from build123d import *

# Parameters (mm, degrees)
SKETCH1_R           = 79.375
SKETCH1_R_2         = 66.675
SKETCH1_R_3         = 1.4224
BOSS_EXTRUDE1_DEPTH = 3.048
SKETCH2_R           = 1.4224
BOSS_EXTRUDE2_DEPTH = 3.048


with BuildPart() as part:
    # Sketch1 → Boss-Extrude1 (new body)
    with BuildSketch(Plane(origin=(0, 0, 0), x_dir=(1, 0, 0), z_dir=(0, 1, 0))):
        with Locations(Location((0, 0, 0), (0, 0, 90))):
            Circle(SKETCH1_R)
        with Locations(Location((0, 0, 0), (0, 0, 90))):
            Circle(SKETCH1_R_2, mode=Mode.SUBTRACT)
        with Locations(Location((0, 73.025, 0), (0, 0, 90))):
            Circle(SKETCH1_R_3, mode=Mode.SUBTRACT)
        with Locations(Location((27.945457648, 67.466302862, 0), (0, 0, 90))):
            Circle(SKETCH1_R_3, mode=Mode.SUBTRACT)
        with Locations(Location((51.636472696, 51.636472696, 0), (0, 0, 90))):
            Circle(SKETCH1_R_3, mode=Mode.SUBTRACT)
        with Locations(Location((67.466302862, 27.945457648, 0), (0, 0, 90))):
            Circle(SKETCH1_R_3, mode=Mode.SUBTRACT)
        with Locations(Location((73.025, 0, 0), (0, 0, 90))):
            Circle(SKETCH1_R_3, mode=Mode.SUBTRACT)
        with Locations(Location((67.466302862, -27.945457648, 0), (0, 0, 90))):
            Circle(SKETCH1_R_3, mode=Mode.SUBTRACT)
        with Locations(Location((51.636472696, -51.636472696, 0), (0, 0, 90))):
            Circle(SKETCH1_R_3, mode=Mode.SUBTRACT)
        with Locations(Location((27.945457648, -67.466302862, 0), (0, 0, 90))):
            Circle(SKETCH1_R_3, mode=Mode.SUBTRACT)
        with Locations(Location((0, -73.025, 0), (0, 0, 90))):
            Circle(SKETCH1_R_3, mode=Mode.SUBTRACT)
        with Locations(Location((-27.945457648, -67.466302862, 0), (0, 0, 90))):
            Circle(SKETCH1_R_3, mode=Mode.SUBTRACT)
        with Locations(Location((-51.636472696, -51.636472696, 0), (0, 0, 90))):
            Circle(SKETCH1_R_3, mode=Mode.SUBTRACT)
        with Locations(Location((-67.466302862, -27.945457648, 0), (0, 0, 90))):
            Circle(SKETCH1_R_3, mode=Mode.SUBTRACT)
        with Locations(Location((-73.025, 0, 0), (0, 0, 90))):
            Circle(SKETCH1_R_3, mode=Mode.SUBTRACT)
        with Locations(Location((-67.466302862, 27.945457648, 0), (0, 0, 90))):
            Circle(SKETCH1_R_3, mode=Mode.SUBTRACT)
        with Locations(Location((-51.636472696, 51.636472696, 0), (0, 0, 90))):
            Circle(SKETCH1_R_3, mode=Mode.SUBTRACT)
        with Locations(Location((-27.945457648, 67.466302862, 0), (0, 0, 90))):
            Circle(SKETCH1_R_3, mode=Mode.SUBTRACT)
    extrude(amount=BOSS_EXTRUDE1_DEPTH)

    # Sketch2 → Boss-Extrude2 (add)
    with BuildSketch(Plane(origin=(0, 3.048, 0), x_dir=(1, 0, 0), z_dir=(0, 1, 0))):
        with BuildLine():
            Line((-15.494, 3.175), (-15.494, 27.813))
            ThreePointArc((-15.494, 27.813), (-12.319, 30.988), (-15.494, 34.163))
            Line((-15.494, 34.163), (-15.494, 58.801))
            ThreePointArc((-15.494, 58.801), (-13.24893597, 59.73093597), (-12.319, 61.976))
            Line((-12.319, 61.976), (-12.319, 65.527077334))
            ThreePointArc((-12.319, 65.527077334), (-17.128346163, 64.437375666), (-21.844, 62.995200524))
            Line((-21.844, 62.995200524), (-21.844, -62.995200524))
            ThreePointArc((-21.844, -62.995200524), (-17.128346163, -64.437375666), (-12.319, -65.527077334))
            Line((-12.319, -65.527077334), (-12.319, -61.976))
            ThreePointArc((-12.319, -61.976), (-13.24893597, -59.73093597), (-15.494, -58.801))
            Line((-15.494, -58.801), (-15.494, -34.163))
            ThreePointArc((-15.494, -34.163), (-12.319, -30.988), (-15.494, -27.813))
            Line((-15.494, -27.813), (-15.494, -3.175))
            ThreePointArc((-15.494, -3.175), (-12.319, 0), (-15.494, 3.175))
        make_face()
        with Locations(Location((-15.494, 30.988, 0), (0, 0, 270))):
            Circle(SKETCH2_R, mode=Mode.SUBTRACT)
        with Locations(Location((-15.494, 0, 0), (0, 0, 270))):
            Circle(SKETCH2_R, mode=Mode.SUBTRACT)
        with Locations(Location((-15.494, 61.976, 0), (0, 0, 270))):
            Circle(SKETCH2_R, mode=Mode.SUBTRACT)
        with Locations(Location((-15.494, -30.988, 0), (0, 0, 270))):
            Circle(SKETCH2_R, mode=Mode.SUBTRACT)
        with Locations(Location((-15.494, -61.976, 0), (0, 0, 270))):
            Circle(SKETCH2_R, mode=Mode.SUBTRACT)
        with BuildLine():
            Line((12.319, 65.527077334), (12.319, 61.976))
            ThreePointArc((12.319, 61.976), (13.24893597, 59.73093597), (15.494, 58.801))
            Line((15.494, 58.801), (15.494, 34.163))
            ThreePointArc((15.494, 34.163), (12.319, 30.988), (15.494, 27.813))
            Line((15.494, 27.813), (15.494, 3.175))
            ThreePointArc((15.494, 3.175), (12.319, 0), (15.494, -3.175))
            Line((15.494, -3.175), (15.494, -27.813))
            ThreePointArc((15.494, -27.813), (12.319, -30.988), (15.494, -34.163))
            Line((15.494, -34.163), (15.494, -58.801))
            ThreePointArc((15.494, -58.801), (13.24893597, -59.73093597), (12.319, -61.976))
            Line((12.319, -61.976), (12.319, -65.527077334))
            ThreePointArc((12.319, -65.527077334), (17.128346163, -64.437375666), (21.844, -62.995200524))
            Line((21.844, -62.995200524), (21.844, 62.995200524))
            ThreePointArc((21.844, 62.995200524), (17.128346163, 64.437375666), (12.319, 65.527077334))
        make_face()
        with Locations(Location((15.494, 61.976, 0), (0, 0, 270))):
            Circle(SKETCH2_R, mode=Mode.SUBTRACT)
        with Locations(Location((15.494, 30.988, 0), (0, 0, 270))):
            Circle(SKETCH2_R, mode=Mode.SUBTRACT)
        with Locations(Location((15.494, -61.976, 0), (0, 0, 270))):
            Circle(SKETCH2_R, mode=Mode.SUBTRACT)
        with Locations(Location((15.494, 0, 0), (0, 0, 270))):
            Circle(SKETCH2_R, mode=Mode.SUBTRACT)
        with Locations(Location((15.494, -30.988, 0), (0, 0, 270))):
            Circle(SKETCH2_R, mode=Mode.SUBTRACT)
    extrude(amount=-BOSS_EXTRUDE2_DEPTH)


solid = part.part
Part model, mm, in its own coordinate system. A direction names the side the tool comes from. Coordinates: 2 decimals unless noted, no trailing zeros. Loops run counter-clockwise (first coordinate to the right, second up) from the corner with the lowest first, then second, coordinate; pieces in that order, holes last. Notation, with made-up numbers: M 49.5,14.5 L 55.5,14.5 A31 ccw 55.5,51.5 Z; hole C -9,-17 d7. An arc over 180 degrees is marked long. Use a Markdown table: item, result. Add a question column.
Q1. Which spindle directions (+Z, -Z, +X, -X, +Y, -Y) get a long thin tool onto all of the face, cutting with end or side? Do faces 1 (the flat face through (17, 3.048, 1)), 2 (the cylindrical face through (-66.665, 1.503, -1.155)). Say none if no direction does.
Q2. Cut at B-B (z = -40.5). Write the cut outline in (x, y), and give its area (3 significant figures).
Q3. Pin check, flat tips, straight feed: P1, Ø0.9, axis at y = 1.5, z = -13.5, coming from the -X side; P2, Ø2.5, axis at x = -15.494, z = 0, coming from the -Y side; P3, Ø1.5, axis at y = 2.5, z = -64, coming from the +X side; P4, Ø1.5, axis at y = 2.5, z = -5, coming from the -X side. Stop position of each tip, or through.
Q4. Mould opens along X. For faces 3 (the flat face through (17, 0, 1)), 4 (the cylindrical face through (-23.84, 1.5, -75.71)), 5 (the cylindrical face through (66.665, 1.503, 1.155)) say: +X half, -X half, draft (parallel to the pull), parting line (faces both ways), or undercut.
Q5. Cut at D-D (z = 11). Write the cut outline in (x, y), and give its area (3 significant figures).
Q6. Cut at A-A (x = -48). Write the cut outline in (y, z), and give its area (3 significant figures).
Q7. Cut at C-C (x = 55.5). Write the cut outline in (y, z), and give its area (3 significant figures).
Q8. Probe L1, parallel to X at y = 2.15, z = -60.5; L2, parallel to X at y = 1.5, z = 35.5; L3, parallel to X at y = 2.25, z = 52. List the from-to ranges inside material, lowest first.
Worked out:
| question | item | result |
|---|---|---|
| 1 | face 1 | +Z, -Z, +X, -X, +Y |
| 1 | face 2 | +Y, -Y |
| 2 | outline | M -68.27,0 L -52.97,0 L -52.97,3.05 L -68.27,3.05 Z; M -21.84,0 L -15.49,0 L -15.49,3.05 L -21.84,3.05 Z; M 15.49,0 L 21.84,0 L 21.84,3.05 L 15.49,3.05 Z; M 52.97,0 L 68.27,0 L 68.27,3.05 L 52.97,3.05 Z |
| 2 | area | 132 mm2 |
| 3 | P1 | stops at x = -78.29 |
| 3 | P2 | passes through |
| 3 | P3 | stops at x = 47.96 |
| 3 | P4 | stops at x = -79.26 |
| 4 | face 3 | draft |
| 4 | face 4 | parting line |
| 4 | face 5 | undercut |
| 5 | outline | M -78.61,0 L -65.76,0 L -65.76,3.05 L -78.61,3.05 Z; M -21.84,0 L -15.49,0 L -15.49,3.05 L -21.84,3.05 Z; M 15.49,0 L 21.84,0 L 21.84,3.05 L 15.49,3.05 Z; M 65.76,0 L 78.61,0 L 78.61,3.05 L 65.76,3.05 Z |
| 5 | area | 117 mm2 |
| 6 | outline | M 0,-63.22 L 3.05,-63.22 L 3.05,-46.28 L 0,-46.28 Z; M 0,46.28 L 3.05,46.28 L 3.05,63.22 L 0,63.22 Z |
| 6 | area | 103 mm2 |
| 7 | outline | M 0,-56.75 L 3.05,-56.75 L 3.05,-36.95 L 0,-36.95 Z; M 0,36.95 L 3.05,36.95 L 3.05,56.75 L 0,56.75 Z |
| 7 | area | 121 mm2 |
| 8 | L1 | x = -51.38 to -28.02, -21.84 to -12.68, 12.68 to 21.84, 28.02 to 51.38 |
| 8 | L2 | x = -70.99 to -56.44, -21.84 to -15.49, 15.49 to 21.84, 56.44 to 70.99 |
| 8 | L3 | x = -59.97 to -53.01, -50.26 to -41.73, -21.84 to -15.49, 15.49 to 21.84, 41.73 to 50.26, 53.01 to 59.97 |
